```python
from build123d import *

# Parameters (mm, degrees)
F0_R     = 10.25
F1_DEPTH = 6
F2_R     = 14.5
F3_DEPTH = 13
F4_R     = 14.5
F5_DEPTH = 10
F6_R     = 9.5
F7_DEPTH = 23


with BuildPart() as f1:
    # F0 (on Front) → F1 (new body)
    with BuildSketch(Plane.XZ):
        Circle(F0_R)
    extrude(amount=F1_DEPTH)

    # F2 (on face) → F3 (join)
    with BuildSketch(Plane.XZ.offset(6)):
        Circle(F2_R)
    extrude(amount=F3_DEPTH)

    # F4 (on face) → F5 (join)
    with BuildSketch(Plane(origin=(0, 0, 0), x_dir=(-1, 0, 0), z_dir=(0, 1, 0))):
        Circle(F4_R)
    extrude(amount=F5_DEPTH)

    # F6 (on face) → F7 (join)
    with BuildSketch(Plane(origin=(0, 10, 0), x_dir=(-1, 0, 0), z_dir=(0, 1, 0))):
        Circle(F6_R)
    extrude(amount=F7_DEPTH)


solid = f1.part
```
Could you check a few things on this model? Use its own coordinates, in mm. A direction names the side the tool comes from. Coordinates: 2 decimals unless noted, no trailing zeros. Write each loop counter-clockwise with the first axis right and the second up, starting at its lowest first coordinate (ties: lowest second). Pieces come first, ordered by that corner, then holes. Notation, with made-up numbers: M 47.25,53.5 L 92.25,53.5 A10 cw 92.25,63.5 Z; hole C 48,82.5 d2. An arc over 180 degrees is marked long. Answer as CSV lines item,"result". Start each with the question number.
1) For P1, Ø6, axis at y = 8.5, z = -4.5, coming from the +X side; P2, Ø5, axis at y = 10, z = 4, coming from the -X side; P3, Ø6, axis at x = 11, y = 22, coming from the +Z side, each with a flat end and sliding along its axis, tell me the tip position at first contact or that it passes through.
2) Please list where these lines run through material, in increasing order: line 1 (Y direction, x = 10.25, z = -10); line 2 (Z direction, x = 0, y = -12); line 3 (Z direction, x = -11.75, y = 4). Write a range as from..to.
3) I want a section at C-C, the plane y = 4.5. Please give me the cut outline in (x, z).
4) I want a section at B-B, the plane z = 4.75. Please give me the cut outline in (x, y).
5) For faces 1 (the cylindrical face through (-6.691, 4.93, -12.864)), 2 (the cylindrical face through (-2.222, -2.958, -10.006)), 3 (the cylindrical face through (-4.38, 21.34, -8.43)), which set-ups out of +Z, -Z, +X, -X, +Y, -Y let a thin tool reach every point of the face, with its end or its side?
6) I want a section at D-D, the plane y = 21. Please give me the cut outline in (x, z), and give its area (3 significant figures).
7) We'd pull the mould along Y, two halves only. Please class faces 4 (the flat face through (-3, 10, -9.5)), 5 (the cylindrical face through (6.691, -12.409, -12.864)), 6 (the flat face through (-3, 0, 10)): +Y half, -Y half, draft (parallel to the pull), parting line (faces both ways), or undercut.
8) I want a section at A-A, the plane x = 0. Please give me the cut outline in (y, z), and give its area (3 significant figures).
Data:
1,P1,"stops at x = 14.42"
1,P2,"stops at x = -14.42"
1,P3,"stops at z = 5.12"
2,line 1,"y = -19..-6, 0..10"
2,line 2,"z = -14.5..14.5"
2,line 3,"z = -8.5..8.5"
3,outline,"C 0,0 d29"
4,outline,"M -13.7,-19 L 13.7,-19 L 13.7,-6 L 9.08,-6 L 9.08,0 L 13.7,0 L 13.7,10 L 8.23,10 L 8.23,33 L -8.23,33 L -8.23,10 L -13.7,10 L -13.7,0 L -9.08,0 L -9.08,-6 L -13.7,-6 Z"
5,face 1,"+Y, -Y"
5,face 2,"none"
5,face 3,"+Y"
6,outline,"C 0,0 d19"
6,area,"284 mm^2"
7,face 4,"+Y half"
7,face 5,"draft"
7,face 6,"undercut"
8,outline,"M -19,-14.5 L -6,-14.5 L -6,-10.25 L 0,-10.25 L 0,-14.5 L 10,-14.5 L 10,-9.5 L 33,-9.5 L 33,9.5 L 10,9.5 L 10,14.5 L 0,14.5 L 0,10.25 L -6,10.25 L -6,14.5 L -19,14.5 Z"
8,area,"1,230 mm^2"
